Build history of the part. All positions in model axes, mm. A direction names the side the tool comes from. Give positions to 0.01 mm unless a question says otherwise; leave off trailing zeros. Loops run counter-clockwise (first coordinate to the right, second up) from the corner with the lowest first, then second, coordinate; pieces in that order, holes last. Notation, with made-up numbers: M -1,24 L 50,24 A11 cw 50,37 Z; hole C -15.75,23 d6. An arc over 180 degrees is marked long. Put each result on its own line as item: value.
Solid Edge part; units mm, degrees
sketch "Sketch1" plane through (0, 0, 0) normal (0, 0, 1) x (1, 0, 0)
  line L0 (0, -30) -> (-180, -30)
  line L1 (-180, -30) -> (-180, 30)
  line L2 (-180, 30) -> (0, 30)
  line L3 (0, 30) -> (0, -30)
extrude "Protrusion1" add sketch "Sketch1" against normal blind 30
sketch "Sketch2" plane through (-90, 0, 0) normal (0, 0, 1) x (1, 0, 0)
  circle A0 centre (-40.5, 11.25) radius 6.35
  circle A1 centre (-40.5, -11.25) radius 6.35
extrude "Recorte_Extrudado_1" cut sketch "Sketch2" against normal blind 30
sketch "Sketch3" plane through (-90, 0, 0) normal (0, 0, 1) x (1, 0, 0)
  line L0 (-34.15, 11.25) -> (-34.15, -11.25)
  line L1 (-34.15, -11.25) -> (-46.85, -11.25)
  line L2 (-46.85, -11.25) -> (-46.85, 11.25)
  line L3 (-46.85, 11.25) -> (-34.15, 11.25)
extrude "Recorte_Extrudado_2" cut sketch "Sketch3" against normal blind 30
chamfer "Chanfro_3" distance 45 angle 45 1 edges at (0, -30, -15)
fillet "Redondo_5" radius 10 2 edges at (0, 30, -15) (0, 15, -15)
fillet "Redondo_6" radius 10 1 edges at (-45, -30, -15)
Q1. Tool access for faces 4 (the flat face through (-114, -30, -15)), 5 (the cylindrical face through (-130.6, -17.6, -14.8)): list every direction of +Z, -Z, +X, -X, +Y, -Y with a clear straight run to the whole face (end or side of a thin tool).
Here are the results:
face 4: +Z, -Z, +X, -X, -Y
face 5: +Z, -Z
Q2. Slice it at D-D (x = -38.5). List the corners of the cut face in (y, z).
Here are the results:
outline: M -23.5,-30 L 30,-30 L 30,0 L -23.5,0 Z
Q3. Slice it at C-C (z = -19.5). List the corners of the cut face in (x, y), and give its area (3 significant figures).
Here are the results:
outline: M -180,-30 L -49.14,-30 A10 ccw -42.07,-27.07 L -2.93,12.07 A10 ccw 0,19.14 L 0,20 A10 ccw -10,30 L -180,30 Z; hole M -136.85,-11.25 A6.35 ccw -124.15,-11.25 L -124.15,11.25 A6.35 ccw -136.85,11.25 Z
area: 9,350 mm²
Q4. Mould opens along X. For faces 1 (the flat face through (-22, -7, -15)), 2 (the flat face through (-136.85, 0, -15)), 3 (the flat face through (-180, 0, -15)) say: pulls with the +X half, pulls with the -X half, needs draft (parallel to the pull), parting line crosses it, or undercut.
Here are the results:
face 1: pulls with the +X half
face 2: undercut
face 3: pulls with the -X half
Q5. Drop flat-ended pins along their axis: pin 1 Ø7 at (y, z) = (-4, -16) entering from +X; pin 2 Ø1.5 at (x, z) = (-18.5, -19.5) entering from -Y. Give the stop position or say it passes through.
Here are the results:
pin 1: x = -15.5
pin 2: y = -4.25
Q6. Slice it at B-B (x = -130.5). List the corners of the cut face in (y, z), and give its area (3 significant figures).
Here are the results:
outline: M -30,-30 L -17.6,-30 L -17.6,0 L -30,0 Z; M 17.6,-30 L 30,-30 L 30,0 L 17.6,0 Z
area: 744 mm²
Q7. Probe line 1 (Y direction, x = -128, z = -8.75); line 2 (X direction, y = -4, z = -15); line 3 (Y direction, x = -49, z = -14.5). List the from-to ranges inside material, lowest first. Write a range as from..to.
Here are the results:
line 1: -30..-17.09, 17.09..30
line 2: -180..-136.85, -124.15..-19
line 3: -30..30
Q8. Slice it at A-A (y = 8). List the corners of the cut face in (x, z).
Here are the results:
outline: M -180,-30 L -136.85,-30 L -136.85,0 L -180,0 Z; M -124.15,-30 L -7,-30 L -7,0 L -124.15,0 Z
